```python
from build123d import *

# Parameters (mm, degrees)
F0_W      = 127
F0_H      = 76.2
F1_DEPTH  = 12.7
F2_R      = 12.7
F3_R      = 12.7
F4_W      = 63.5
F4_H      = 25.4
F5_DEPTH  = 63.5
F7_DEPTH  = 25.4
F8_DEPTH  = 25.4
F9_R      = 20.636463447
F11_DEPTH = 25.4010001
F12_DEPTH = 25.4010001
F13_R     = 0.2708197303
F14_R     = 6.35
F15_DEPTH = 12.7010001
F16_DEPTH = 12.7010001
F17_DEPTH = 12.7010001


with BuildPart() as f1:
    # F0 (on Top) → F1 (new body)
    with BuildSketch(Plane.XY):
        with Locations((1.7509019642, 4.0471330285)):
            Rectangle(F0_W, F0_H)
    extrude(amount=F1_DEPTH)

    # F2
    f2_edges = [f1.edges().sort_by_distance(p)[0] for p in [
        (-61.749098, -34.052867, 6.35),
    ]]
    fillet(f2_edges, radius=F2_R)

    # F3
    f3_edges = [f1.edges().sort_by_distance(p)[0] for p in [
        (65.250902, -34.052867, 6.35),
    ]]
    fillet(f3_edges, radius=F3_R)

    # F4 (on face) → F5 (join)
    with BuildSketch(Plane.XY.offset(12.7)):
        with Locations((-29.9990980358, 29.4471330285)):
            Rectangle(F4_W, F4_H)
    extrude(amount=F5_DEPTH)

    # F6 (on face) → F7 (join)
    with BuildSketch(Plane.XZ.offset(-16.7471330285)):
        with BuildLine():
            Line((-61.7490980358, 76.2), (1.7509019642, 76.2))
            ThreePointArc((1.7509019642, 76.2), (-29.9990980358, 94.2832173296), (-61.7490980358, 76.2))
        make_face()
    extrude(amount=-F7_DEPTH)

    # F6 (on face) → F8 (join)
    with BuildSketch(Plane.XZ.offset(-16.7471330285)):
        with BuildLine():
            ThreePointArc((26.2496182163, 12.7), (8.0879587681, 42.1689953939), (1.7509019642, 76.2))
            Line((1.7509019642, 76.2), (1.7509019642, 12.7))
            Line((1.7509019642, 12.7), (26.2496182163, 12.7))
        make_face()
    extrude(amount=-F8_DEPTH)

    # F9
    f9_edges = [f1.edges().sort_by_distance(p)[0] for p in [
        (1.750902, 29.447133, 76.2),
    ]]
    fillet(f9_edges, radius=F9_R)

    # F10 (on face) → F11 (cut, through all)
    with BuildSketch(Plane.XZ.offset(-16.7471330285)):
        with BuildLine():
            ThreePointArc((-40.1649535069, 76.2), (-33.624820371, 56.7753634634), (-17.0858500555, 68.8812424863))
            ThreePointArc((-17.0858500555, 68.8812424863), (-17.6799710326, 72.7202128018), (-19.4067466041, 76.2))
            Line((-19.4067466041, 76.2), (-40.1649535069, 76.2))
        make_face()
    extrude(amount=-F11_DEPTH, mode=Mode.SUBTRACT)

    # F10 (on face) → F12 (cut, through all)
    with BuildSketch(Plane.XZ.offset(-16.7471330285)):
        with BuildLine():
            Line((-40.1649535069, 76.2), (-19.4067466041, 76.2))
            ThreePointArc((-19.4067466041, 76.2), (-29.7858500555, 81.5812424863), (-40.1649535069, 76.2))
        make_face()
    extrude(amount=-F12_DEPTH, mode=Mode.SUBTRACT)

    # F13
    f13_edges = [f1.edges().sort_by_distance(p)[0] for p in [
        (-61.749098, 29.447133, 76.2),
    ]]
    fillet(f13_edges, radius=F13_R)

    # F14 (on face) → F15 (cut, through all)
    with BuildSketch(Plane.XY.offset(12.7)):
        with Locations((-41.6999144272, -15.0028669715)):
            Circle(F14_R)
    extrude(amount=-F15_DEPTH, mode=Mode.SUBTRACT)

    # F14 (on face) → F16 (cut, through all)
    with BuildSketch(Plane.XY.offset(12.7)):
        with Locations((46.2009019642, -15.0028669715)):
            Circle(F14_R)
    extrude(amount=-F16_DEPTH, mode=Mode.SUBTRACT)

    # F14 (on face) → F17 (cut, through all)
    with BuildSketch(Plane.XY.offset(12.7)):
        with Locations((46.2009019642, 23.1024639082)):
            Circle(F14_R)
    extrude(amount=-F17_DEPTH, mode=Mode.SUBTRACT)


solid = f1.part
```
The listing builds one solid part. Answer for the finished solid, in the listing's coordinates (mm). A direction names the side the tool comes from. Coordinates: 2 decimals unless noted, no trailing zeros. Loops run counter-clockwise (first coordinate to the right, second up) from the corner with the lowest first, then second, coordinate; pieces in that order, holes last. Notation, with made-up numbers: M -23,-4.75 L 29,-4.75 A24 ccw 29,6.25 Z; hole C -30.75,13 d9. An arc over 180 degrees is marked long. Answer as a JSON object with one key per item and string values. Group by question number.
Item 1: Section C-C (x = 46) is taken. Write down the section's boundary in (y, z).
Item 2: Which of the six approach directions +Z, -Z, +X, -X, +Y, -Y give full straight-line access (tool end or side, diameter ignored) to faces 1 (the face through (-13, 42.147, 37)), 2 (the face through (-28, 16.747, 45)), 3 (the face through (1, -4, 12.7))?
Item 3: Determine the mould class of faces 4 (the face through (1, 5, 0)), 5 (the face through (65.251, 10, 6)), 6 (the face through (44.82, -21.2, 6.44)) for opening direction X: +X half, -X half, draft (parallel to the pull), parting line (faces both ways), or undercut.
Item 4: Each of these flat-tipped pins is pushed along its axis until it touches: P1, Ø6, axis at x = -8.5, z = 58, coming from the -Y side; P2, Ø6, axis at x = 29, y = -1.5, coming from the +Z side. Where does it stop, or does it pass through?
Item 5: Section B-B (y = 19.5) is taken. Give the number of separate pieces and of enclosed holes in the cut face, and give its area (3 significant figures).
Item 6: Consider L1, parallel to Y at x = -3, z = 14; L2, parallel to Z at x = -16, y = -28; L3, parallel to X at y = -11.5, z = 10.5. Determine where each line is inside the solid, lowest interval first.
Item 7: Section D-D (z = 35) is taken. Write down the section's boundary in (x, y).
Item 8: Section A-A (x = -25) is taken. Write down the section's boundary in (y, z), and give its area (3 significant figures).
Solved:
{
 "1": {"outline": "M -34.05,0 L -21.35,0 L -21.35,12.7 L -34.05,12.7 Z; M -8.66,0 L 16.76,0 L 16.76,12.7 L -8.66,12.7 Z; M 29.45,0 L 42.15,0 L 42.15,12.7 L 29.45,12.7 Z"},
 "2": {"face 1": "+Z, -Z, +X, -X, +Y", "face 2": "+Z, +X, -X, -Y", "face 3": "+Z, +X, -Y"},
 "3": {"face 4": "draft", "face 5": "+X half", "face 6": "undercut"},
 "4": {"P1": "stops at y = 16.75", "P2": "stops at z = 12.7"},
 "5": {"separate pieces": "2", "enclosed holes": "1", "area": "6,300 mm2"},
 "6": {"L1": "y = 16.75 to 42.15", "L2": "z = 0 to 12.7", "L3": "x = -61.75 to -47, -36.4 to 40.9, 51.5 to 65.25"},
 "7": {"outline": "M -61.75,16.75 L 11.2,16.75 L 11.2,42.15 L -61.75,42.15 Z"},
 "8": {"outline": "M -34.05,0 L 42.15,0 L 42.15,57.12 L 16.75,57.12 L 16.75,12.7 L -34.05,12.7 Z; M 16.75,80.64 L 42.15,80.64 L 42.15,93.94 L 16.75,93.94 Z", "area": "2,430 mm2"}
}
